Here's the drawing with two shaded views (mm, measured from the low corner). I have some questions. A direction names the side the tool comes from. Coordinates: 2 decimals unless noted, no trailing zeros. Loops run counter-clockwise (first coordinate to the right, second up) from the corner with the lowest first, then second, coordinate; pieces in that order, holes last.
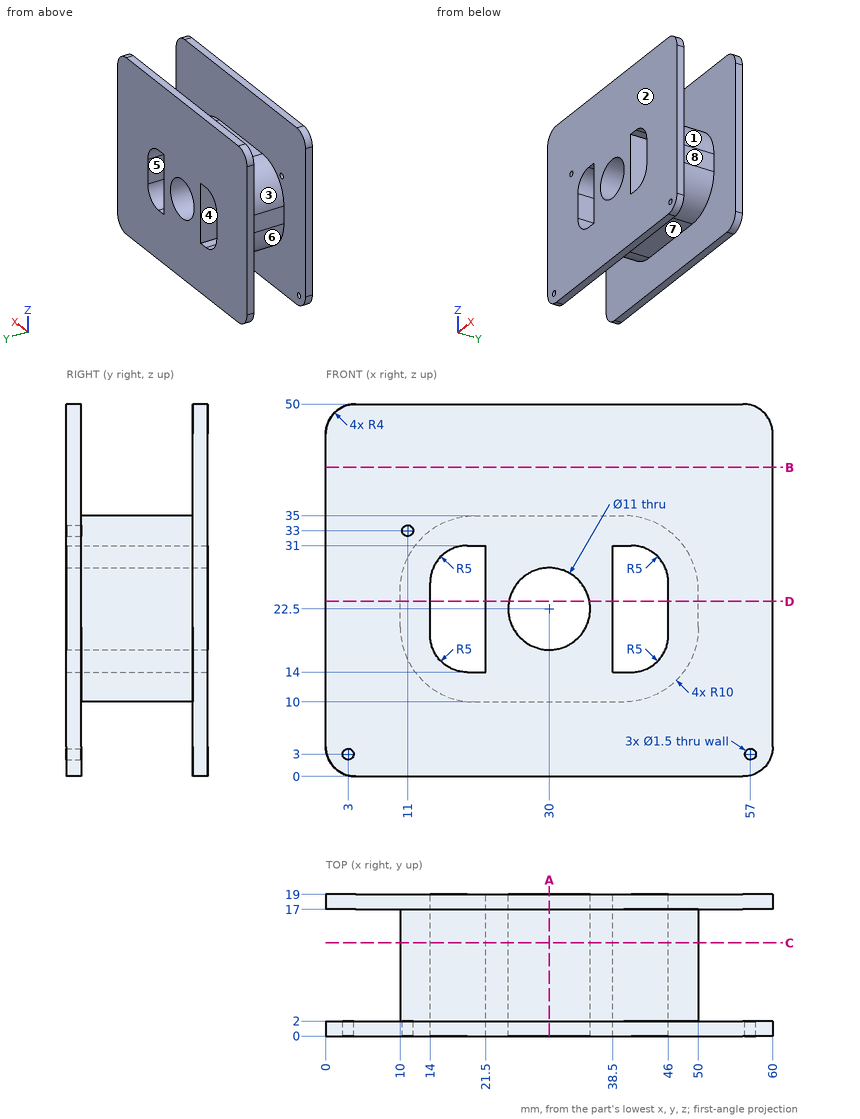
(1) I'm going to push flat-ended pins straight in: pin 1 (6 mm diameter, centred on y = 9.5, z = 40, fed in from -X); pin 2 (5 mm diameter, centred on y = 6.5, z = 21.5, fed in from -X); pin 3 (4 mm diameter, centred on y = 11.5, z = 23, fed in from +X); pin 4 (8 mm diameter, centred on y = 11.5, z = 10, fed in from -X). Where does each tip first touch, or does it pass through?
Check values:
pin 1: passes through
pin 2: stops at x = 10
pin 3: stops at x = 50
pin 4: stops at x = 12
(2) If I drill on probe 1 along Y at (x, z) = (36.5, 8); probe 2 along X at (y, z) = (1.45, 33); probe 3 along X at (y, z) = (13, 12), over which ranges is the centre line in solid material (lowest first)?
Check values:
probe 1: y = 0 to 2, 17 to 19
probe 2: x = 0 to 10.25, 11.75 to 60
probe 3: x = 14 to 46
(3) Which directions (+Z, -Z, +X, -X, +Y, -Y) give clear straight access to the entire face, cutting with the end or side of a thin tool? Please do the marked faces 5, 6, 7 and 8.
Check values:
face 5: +Y, -Y
face 6: -Z, -X
face 7: -Z, +X, -X
face 8: +Z, -Z, +X
(4) I want a section at D-D on z = 23.5. Write out the boundary of the cut face in (x, y).
Check values:
outline: (0, 0) - (14, 0) - (14, 19) - (0, 19) - (0, 17) - (10, 17) - (10, 2) - (0, 2) - close; (21.5, 0) - (24.59, 0) - (24.59, 19) - (21.5, 19) - close; (35.41, 0) - (38.5, 0) - (38.5, 19) - (35.41, 19) - close; (46, 0) - (60, 0) - (60, 2) - (50, 2) - (50, 17) - (60, 17) - (60, 19) - (46, 19) - close
(5) I want a section at C-C on y = 12.5. Write out the boundary of the cut face in (x, z), then the cut area to 3 significant figures.
Check values:
outline: (10, 20) arc R10 ccw to (20, 10) - (40, 10) arc R10 ccw to (50, 20) - (50, 25) arc R10 ccw to (40, 35) - (20, 35) arc R10 ccw to (10, 25) - close; hole (14, 19) arc R5 ccw to (19, 14) - (21.5, 14) - (21.5, 31) - (19, 31) arc R5 ccw to (14, 26) - close; hole circle Ø11 at (30, 22.5); hole (38.5, 14) - (41, 14) arc R5 ccw to (46, 19) - (46, 26) arc R5 ccw to (41, 31) - (38.5, 31) - close
area: 586 mm2
(6) I want a section at A-A on x = 30. Write out the boundary of the cut face in (y, z), then the cut area to 3 significant figures.
Check values:
outline: (0, 0) - (2, 0) - (2, 10) - (17, 10) - (17, 0) - (19, 0) - (19, 17) - (0, 17) - close; (0, 28) - (19, 28) - (19, 50) - (17, 50) - (17, 35) - (2, 35) - (2, 50) - (0, 50) - close
area: 366 mm2
(7) I want a section at B-B on z = 41.5. Write out the boundary of the cut face in (x, y).
Check values:
outline: (0, 0) - (60, 0) - (60, 2) - (0, 2) - close; (0, 17) - (60, 17) - (60, 19) - (0, 19) - close
(8) If we mould it in two halves opening along X, with no side actions, what happens to the marked faces 1, 2, 3 and 4? For each: released by +X, released by -X, zero draft, split by the parting line, or undercut.
Check values:
face 1: released by +X
face 2: zero draft
face 3: released by -X
face 4: undercut
